```python
from build123d import *

# Parameters (mm, degrees)
SKETCH_W        = 73
SKETCH_H        = 19
PAD_DEPTH       = 5
SKETCH001_W     = 69
SKETCH001_H     = 3
POCKET_DEPTH    = 5.001
SKETCH002_W     = 69
SKETCH002_H     = 3
POCKET001_DEPTH = 19.001
POCKET002_DEPTH = 2.001


with BuildPart() as part:
    # Sketch → Pad (new body)
    with BuildSketch(Plane.XY):
        Rectangle(SKETCH_W, SKETCH_H)
    extrude(amount=PAD_DEPTH)

    # Sketch001 → Pocket (cut, through all)
    with BuildSketch(Plane.XY.offset(5)):
        with Locations((-2, 8)):
            Rectangle(SKETCH001_W, SKETCH001_H)
        with Locations((-2, -8)):
            Rectangle(SKETCH001_W, SKETCH001_H)
    extrude(amount=-POCKET_DEPTH, mode=Mode.SUBTRACT)

    # Sketch002 → Pocket001 (cut, through all)
    with BuildSketch(Plane.XZ.offset(9.5)):
        with Locations((2, 3.5)):
            Rectangle(SKETCH002_W, SKETCH002_H)
    extrude(amount=-POCKET001_DEPTH, mode=Mode.SUBTRACT)

    # Sketch003 → Pocket002 (cut, through all)
    with BuildSketch(Plane.XY.offset(2)):
        with BuildLine():
            Line((-1.5, 5), (36.5, 5))
            Line((36.5, 5), (36.5, -5))
            Line((36.5, -5), (-1.5, -5))
            ThreePointArc((-1.5, 5), (-6.5, 0), (-1.5, -5))
        make_face()
    extrude(amount=-POCKET002_DEPTH, mode=Mode.SUBTRACT)


solid = part.part
```
Read the model definition and answer for the solid it produces. Units are mm, in the model's axes. A direction names the side the tool comes from. Give positions to 0.01 mm unless a question says otherwise; leave off trailing zeros. Write each loop counter-clockwise with the first axis right and the second up, starting at its lowest first coordinate (ties: lowest second). Pieces come first, ordered by that corner, then holes. Notation, with made-up numbers: (51, 55.5) -> (89, 55.5) arc R33 cw to (89, 84.5) -> close; hole circle Ø5 at (76.5, 89.5). An arc over 180 degrees is marked (long way). Answer in a Markdown table with one row per item.
1) Each of these flat-tipped pins is pushed along its axis until it touches: pin 1 Ø3 at (y, z) = (0, 1) entering from +X; pin 2 Ø2 at (x, z) = (24.5, 0.5) entering from +Y; pin 3 Ø8 at (x, y) = (-27, 0) entering from -Z; pin 4 Ø1.6 at (x, z) = (17.5, 1.5) entering from -Y. Where does it stop, or does it pass through?
Results list:
| item | result |
|---|---|
| pin 1 | x = -6.27 |
| pin 2 | y = 6.5 |
| pin 3 | z = 0 |
| pin 4 | y = -6.5 |
2) Section A-A on x = -5.5 is taken. Give the vertices of the cut face in (y, z), plus the area to 3 significant figures.
Results list:
| item | result |
|---|---|
| outline | (-6.5, 0) -> (-3, 0) -> (-3, 2) -> (-6.5, 2) -> close; (3, 0) -> (6.5, 0) -> (6.5, 2) -> (3, 2) -> close |
| area | 14.0 mm^2 |
3) A tool of negligible diameter and unlimited length cuts with its end or side. For faces 1 (the flat face through (-2, 6.5, 1)), 2 (the flat face through (-32.5, 0, 3)), 3 (the flat face through (18, -5, 1)), 4 (the flat face through (32.5, -8, 1)), from which of +Z, -Z, +X, -X, +Y, -Y can it reach the whole face along a straight path? Write none if from no direction.
Results list:
| item | result |
|---|---|
| face 1 | +Z, -Z, -X, +Y |
| face 2 | +Z, +X, +Y, -Y |
| face 3 | +Z, -Z, +X |
| face 4 | +Z, -Z, -X, -Y |
4) Section C-C on y = -7.75 is taken. Give the vertices of the cut face in (x, z), plus the area to 3 significant figures.
Results list:
| item | result |
|---|---|
| outline | (32.5, 0) -> (36.5, 0) -> (36.5, 2) -> (32.5, 2) -> close |
| area | 8.00 mm^2 |
5) Straight lines are drawn through the part: line 1 (Y direction, x = 29, z = 1.35); line 2 (X direction, y = -2.25, z = 3.95); line 3 (Z direction, x = -31, y = -4). For each, find the intervals that lie inside material, in ascending order. Write a range as [from, to].
Results list:
| item | result |
|---|---|
| line 1 | [-6.5, -5], [5, 6.5] |
| line 2 | [-36.5, -32.5] |
| line 3 | [0, 2] |
6) Section B-B on x = 4.5 is taken. Give the vertices of the cut face in (y, z), plus the area to 3 significant figures.
Results list:
| item | result |
|---|---|
| outline | (-6.5, 0) -> (-5, 0) -> (-5, 2) -> (-6.5, 2) -> close; (5, 0) -> (6.5, 0) -> (6.5, 2) -> (5, 2) -> close |
| area | 6.00 mm^2 |
7) Section D-D on x = -16 is taken. Give the vertices of the cut face in (y, z).
Results list:
| item | result |
|---|---|
| outline | (-6.5, 0) -> (6.5, 0) -> (6.5, 2) -> (-6.5, 2) -> close |
